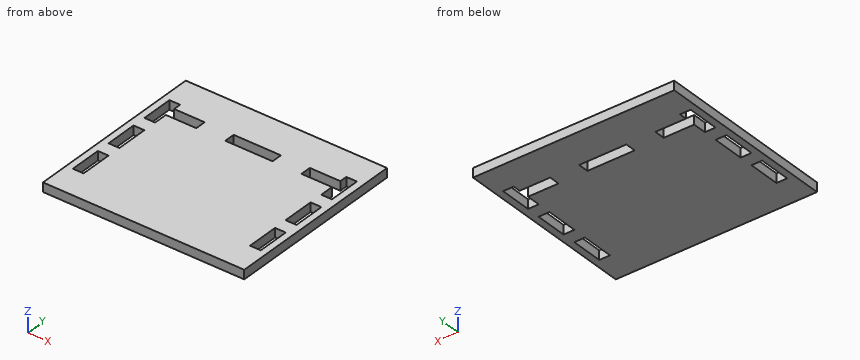
from build123d import *

# Parameters (mm, degrees)
SKETCH_1_W      = 66
SKETCH_1_H      = 60
SKETCH_1_W_2    = 15.5
SKETCH_1_H_2    = 3.5
SKETCH_1_W_3    = 3.566819074
SKETCH_1_H_3    = 10.5
SKETCH_1_W_4    = 3.520169939
EXTRUDE_1_DEPTH = 3


with BuildPart() as part:
    # Эскиз1 → Бобышка-Вытянуть1 (new body)
    with BuildSketch(Plane.XY):
        Rectangle(SKETCH_1_W, SKETCH_1_H)
        with Locations((0, 16)):
            Rectangle(SKETCH_1_W_2, SKETCH_1_H_2, mode=Mode.SUBTRACT)
        Polygon((-17.25, 17.75), (-27.25, 17.75), (-27.25, 20.25), (-30.75, 20.25), (-30.75, 9.75), (-27.25, 9.75), (-27.25, 14.25), (-17.25, 14.25), align=None, mode=Mode.SUBTRACT)
        with Locations((-29.033409537, 0)):
            Rectangle(SKETCH_1_W_3, SKETCH_1_H_3, mode=Mode.SUBTRACT)
        with Locations((-29.056734105, -15)):
            Rectangle(SKETCH_1_W_4, SKETCH_1_H_3, mode=Mode.SUBTRACT)
        with Locations((29.056734105, -15)):
            Rectangle(SKETCH_1_W_4, SKETCH_1_H_3, mode=Mode.SUBTRACT)
        with Locations((29.033409537, 0)):
            Rectangle(SKETCH_1_W_3, SKETCH_1_H_3, mode=Mode.SUBTRACT)
        Polygon((27.25, 20.25), (27.25, 17.75), (17.25, 17.75), (17.25, 14.25), (27.25, 14.25), (27.25, 9.75), (30.75, 9.75), (30.75, 20.25), align=None, mode=Mode.SUBTRACT)
    extrude(amount=EXTRUDE_1_DEPTH)


solid = part.part
Model file for the job. Use its own axes, mm. Give positions to 0.01 mm unless a question says otherwise; leave off trailing zeros. Order: outer loops, then holes, each group sorted by start corner. A loop starts at its lowest first (then second) coordinate and runs counter-clockwise, first axis right, second up. Notation, with made-up numbers: M -26.75,69 L 6.25,69 A27 cw 6.25,94 Z; hole C 32.5,38.25 d10. An arc over 180 degrees is marked long. Put each result on its own line as item: value. Start each with the question number.
(1) Drill centre lines: L1, parallel to X at y = 12.5, z = 1.25; L2, parallel to X at y = -19, z = 1.7; L3, parallel to Y at x = 30, z = 2.5. Where is each one in solid material? Low to high. Write a range as [from, to].
(2) Band-saw the part on C-C on y = 17. Give the cut face in (x, z).
(3) Band-saw the part on D-D on z = 2.3. Count the separate pieces of the cut face and the enclosed holes in it, then the cut area to 3 significant figures.
(4) Band-saw the part on A-A on y = -11.5. Give the cut face in (x, z), then the cut area to 3 significant figures.
(5) Band-saw the part on B-B on x = 0.5. Give the cut face in (y, z).
Results below:
1. L1: x = [-33, -30.75], [-27.25, 27.25], [30.75, 33]
1. L2: x = [-33, -30.82], [-27.3, 27.3], [30.82, 33]
1. L3: y = [-30, -20.25], [-9.75, -5.25], [5.25, 9.75], [20.25, 30]
2. outline: M -33,0 L -30.75,0 L -30.75,3 L -33,3 Z; M -17.25,0 L -7.75,0 L -7.75,3 L -17.25,3 Z; M 7.75,0 L 17.25,0 L 17.25,3 L 7.75,3 Z; M 30.75,0 L 33,0 L 33,3 L 30.75,3 Z
3. separate pieces: 1
3. enclosed holes: 7
3. area: 3,610 mm2
4. outline: M -33,0 L -30.82,0 L -30.82,3 L -33,3 Z; M -27.3,0 L 27.3,0 L 27.3,3 L -27.3,3 Z; M 30.82,0 L 33,0 L 33,3 L 30.82,3 Z
4. area: 177 mm2
5. outline: M -30,0 L 14.25,0 L 14.25,3 L -30,3 Z; M 17.75,0 L 30,0 L 30,3 L 17.75,3 Z
